from build123d import *

# Parameters (mm, degrees)
F1_DEPTH = 5
F2_R     = 1.074979


with BuildPart() as f1:
    # F0 (on Top) → F1 (new body)
    with BuildSketch(Plane.XY):
        with BuildLine():
            Line((18.290205, 33.941125), (-15.65092, 0))
            ThreePointArc((-15.65092, 0), (1.319643, 4.121436), (18.290205, 0))
            ThreePointArc((18.290205, 0), (14.16877, 16.970563), (18.290205, 33.941125))
        make_face()
    extrude(amount=F1_DEPTH)

    # F2
    f2_edges = [f1.edges().sort_by_distance(p)[0] for p in [
        (18.290205, 33.941125, 2.5),
        (-15.65092, 0, 2.5),
        (18.290205, 0, 2.5),
    ]]
    fillet(f2_edges, radius=F2_R)


solid = f1.part
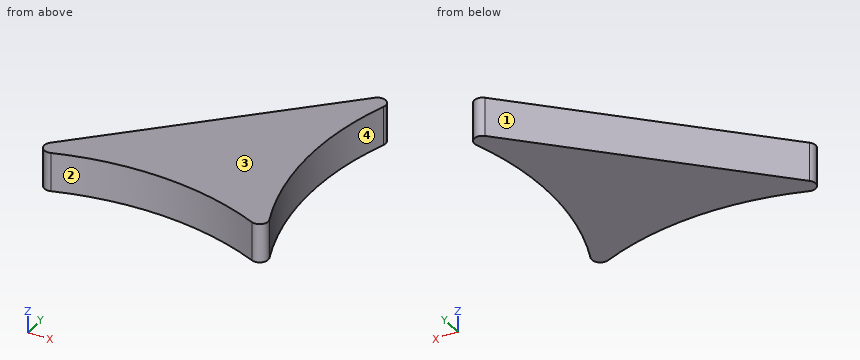
Build history of the part. All positions in model axes, mm. Face numbers are marked on the shaded views. Round coordinates to 2 decimals unless told otherwise and drop trailing zeros. Loops run counter-clockwise (first coordinate to the right, second up) from the corner with the lowest first, then second, coordinate; pieces in that order, holes last. Notation, with made-up numbers: (87, 22.25) -> (123, 22.25) arc R15 ccw to (123, 36.25) -> close; hole circle Ø11 at (36.5, 85.25). An arc over 180 degrees is marked (long way). Use CSV: the item, a comma, the result in double quotes. Start each with the question number.
Q1. Saw through at C-C on y = 14.25. Give the cut face in (x, z), and give its area (3 significant figures).
Q2. Flat gauge pins, fed straight in: pin 1 Ø1 at (y, z) = (4, 1) entering from -X; pin 2 Ø1.5 at (x, z) = (-6.5, 1) entering from -Y. Where does each tip first touch, or does it go through?
Q3. Saw through at B-B on x = -4.25. Give the cut face in (y, z), and give its area (3 significant figures).
Q4. Mould opens along X. For the marked faces 1, 2, 3 and 4 say: +X half, -X half, draft (parallel to the pull), parting line (faces both ways), or undercut.
Q5. Saw through at A-A on y = 3.5. Give the cut face in (x, z).
Q6. Drill centre lines: L1, parallel to Y at x = 4, z = 3.4; L2, parallel to X at y = 28.25, z = 4.4; L3, parallel to X at y = 5, z = 1.25. Where is each one in solid material? Low to high.
Solutions:
1,outline,"(-1.4, 0) -> (14.27, 0) -> (14.27, 5) -> (-1.4, 5) -> close"
1,area,"78.3 mm^2"
2,pin 1,"stops at x = -11.99"
2,pin 2,"stops at y = 3.12"
3,outline,"(3.7, 0) -> (11.4, 0) -> (11.4, 5) -> (3.7, 5) -> close"
3,area,"38.5 mm^2"
4,face 1,"-X half"
4,face 2,"undercut"
4,face 3,"draft"
4,face 4,"+X half"
5,outline,"(-11.99, 0) -> (-5.43, 0) -> (-5.43, 5) -> (-11.99, 5) -> close; (8.07, 0) -> (16.71, 0) -> (16.71, 5) -> (8.07, 5) -> close"
6,L1,"y = 4.02 to 19.65"
6,L2,"x = 12.6 to 15.93"
6,L3,"x = -10.65 to 16.16"
